```python
from build123d import *

# Parameters (mm, degrees)
CUT_EXTRUDE1_REACH = 76.623


with BuildPart() as part:
    # Sketch1 → Revolve1 (revolve)
    with BuildSketch(Plane.XY, mode=Mode.PRIVATE) as revolve1_sk:
        Polygon((31.75, 9.652), (0, 9.652), (0, 15.875), (3.175, 15.875), (3.175, 47.752), (7.62, 47.752), (12.7, 36.6395), (22.225, 36.6395), (27.305, 47.752), (31.75, 47.752), align=None)
    revolve(revolve1_sk.sketch.rotate(Axis((0, 0, 0), (1, 0, 0)), 90), axis=Axis((0, 0, 0), (1, 0, 0)))

    # Sketch2 → Cut-Extrude1 (cut, up to next)
    with BuildSketch(Plane.ZY, mode=Mode.PRIVATE) as cut_extrude1_sk1:
        with BuildLine():
            Line((-2.4384, 9.338913718), (-2.4384, 11.811))
            Line((-2.4384, 11.811), (2.4384, 11.811))
            Line((2.4384, 11.811), (2.4384, 9.338913718))
            ThreePointArc((2.4384, 9.338913718), (0, 9.652), (-2.4384, 9.338913718))
        make_face()
    cut_extrude1_tool1 = extrude(cut_extrude1_sk1.sketch, amount=-CUT_EXTRUDE1_REACH, mode=Mode.PRIVATE) & part.part
    add(cut_extrude1_tool1.solids().sort_by_distance((0, 10.677746, 0))[0], mode=Mode.SUBTRACT)


solid = part.part
```
Input: part model. Units: mm. Frame: model coordinates. A direction names the side the tool comes from. Coordinates: 2 decimals unless noted, no trailing zeros. Write each loop counter-clockwise with the first axis right and the second up, starting at its lowest first coordinate (ties: lowest second). Pieces come first, ordered by that corner, then holes. Notation, with made-up numbers: (13, 38) -> (25, 38) arc R23 ccw to (25, 68) -> close; hole circle Ø11 at (-31.5, 89). An arc over 180 degrees is marked (long way). Answer as a JSON object with one key per item and string values.
1. Section C-C on x = 6.5. Return the cut outline in (y, z).
Result set:
{"outline": "circle Ø95.5 at (0, 0); hole (9.34, -2.44) -> (11.81, -2.44) -> (11.81, 2.44) -> (9.34, 2.44) arc R9.65 ccw (long way) to start"}
2. First-contact query: P1, Ø10, axis at y = 30.5, z = 34, coming from the -X side (3 decimals); P2, Ø8, axis at x = 11.5, z = -10.5, coming from the -Y side; P3, Ø2, axis at x = 11.5, y = 11, coming from the -Z side. Flat tips, straight axial feed; report the tip coordinate or a pass-through.
Result set:
{"P1": "stops at x = 3.175", "P2": "stops at y = -46.79", "P3": "stops at z = -39.98"}
3. Material intervals for line 1 (Y direction, x = 13, z = 0); line 2 (X direction, y = -11.5, z = 13.5) (3 decimals); line 3 (X direction, y = -39.5, z = 11) (3 decimals), sorted ascending. Write a range as from..to.
Result set:
{"line 1": "y = -36.64..-9.65, 11.81..36.64", "line 2": "x = 3.175..31.75", "line 3": "x = 3.175..10.705, 24.22..31.75"}
4. Access query for faces 1 (the face through (0, 7, -7)), 2 (the face through (17.529, -11.006, 34.948)), 3 (the face through (16, 11.811, 0)), 4 (the face through (1.61, 15.497, -3.441)). Directions: +Z, -Z, +X, -X, +Y, -Y. A direction counts if a zero-diameter tool reaches every point of the face in a straight line with its end or side. Return the directions, or none.
Result set:
{"face 1": "+Z, -Z, -X, +Y, -Y", "face 2": "none", "face 3": "+X, -X", "face 4": "-X"}
5. Mould query, pull axis Y, two halves, no side actions, for faces 5 (the face through (22.543, -37.017, -4.86)), 6 (the face through (31.75, -1, 10)), 7 (the face through (15.653, -9.644, 0.39)). Classes: released by +Y, released by -Y, zero draft, split by the parting line, or undercut.
Result set:
{"face 5": "split by the parting line", "face 6": "zero draft", "face 7": "undercut"}
6. Section D-D on x = 14.5. Return the cut outline in (y, z), then the cut area to 3 significant figures.
Result set:
{"outline": "circle Ø73.28 at (0, 0); hole (9.34, -2.44) -> (11.81, -2.44) -> (11.81, 2.44) -> (9.34, 2.44) arc R9.65 ccw (long way) to start", "area": "3,910 mm2"}
